Input: part model. Units: mm. Frame: model coordinates. A direction names the side the tool comes from. Give positions to 0.01 mm unless a question says otherwise; leave off trailing zeros. Write each loop counter-clockwise with the first axis right and the second up, starting at its lowest first coordinate (ties: lowest second). Pieces come first, ordered by that corner, then holes. Notation, with made-up numbers: (22, 76) -> (60, 76) arc R17 cw to (60, 81) -> close; hole circle Ø4 at (-27.75, 52.5). An arc over 180 degrees is marked (long way). Return JSON: item names as keys, results as strings. Group by question number.
Item 1: Line query: line 1 (Y direction, x = 0, z = 90); line 2 (Y direction, x = 0, z = -3); line 3 (X direction, y = -0.5, z = 57.5) (3 decimals). Output: solid intervals per line, ascending. Write a range as [from, to].
Item 2: Pin query (flat end, axial travel): P1, Ø5, axis at x = 0, y = 0, coming from the +Z side; P2, Ø1.3, axis at x = 0.5, y = 20.5, coming from the +Z side; P3, Ø2, axis at x = 12.5, z = 47, coming from the +Y side; P4, Ø1.5, axis at y = -4.5, z = 69, coming from the +X side. Return the tip coordinate at first contact, or that it passes through.
Item 3: Section B-B, the plane y = 0. Return loops of the section in (x, z).
Item 4: Mould query, pull axis Y, two halves, no side actions, for faces 3 (the face through (23.846, -7.509, 45.345)), 4 (the face through (0, 5, -5)), 5 (the face through (17, -10, 76.3)). Classes: released by +Y, released by -Y, zero draft, split by the parting line, or undercut.
Item 5: Section A-A, the plane x = 0. Return loops of the section in (y, z), then the cut area to 3 significant figures.
Item 6: Section C-C, the plane y = 20. Return loops of the section in (x, z).
Item 7: Set-up query: faces 1 (the face through (1.43, 2.75, -2.54)), 2 (the face through (-17, 10, 76.3)). Return all of +Z, -Z, +X, -X, +Y, -Y with unobstructed straight access to the full face (end or side cutting, diameter ignored); none if empty.
Item 8: Section D-D, the plane z = 62.5. Return loops of the section in (x, y), then the cut area to 3 significant figures.
from build123d import *

# Parameters (mm, degrees)
F0_R     = 25
F0_R_2   = 15
F1_DEPTH = 94.3
F2_R     = 2.25
F3_DEPTH = 18
F4_R     = 25
F5_DEPTH = 5
F6_R     = 3.1
F7_DEPTH = 25


with BuildPart() as f1:
    # F0 (on Top) → F1 (new body)
    with BuildSketch(Plane.XY):
        Circle(F0_R)
        Circle(F0_R_2, mode=Mode.SUBTRACT)
    extrude(amount=F1_DEPTH)

    # F2 (on face) → F3 (cut)
    with BuildSketch(Plane.XY.offset(94.3)):
        with Locations((0, 20)):
            Circle(F2_R)
        with Locations((-17.320508, -10)):
            Circle(F2_R)
        with Locations((17.320508, -10)):
            Circle(F2_R)
        with Locations((0, -20)):
            Circle(F2_R)
        with Locations((17.320508, 10)):
            Circle(F2_R)
        with Locations((-17.320508, 10)):
            Circle(F2_R)
    extrude(amount=-F3_DEPTH, mode=Mode.SUBTRACT)

    # F4 (on face) → F5 (join)
    with BuildSketch(Plane(origin=(0, 0, 0), x_dir=(1, 0, 0), z_dir=(0, 0, -1))):
        Circle(F4_R)
    extrude(amount=F5_DEPTH)

    # F6 (on face) → F7 (cut)
    with BuildSketch(Plane(origin=(0, 0, -5), x_dir=(1, 0, 0), z_dir=(0, 0, -1))):
        Circle(F6_R)
    extrude(amount=-F7_DEPTH, mode=Mode.SUBTRACT)


solid = f1.part
Answer below:
{
 "1": {"line 1": "y = [-25, -22.25], [-17.75, -15], [15, 17.75], [22.25, 25]", "line 2": "y = [-25, -3.1], [3.1, 25]", "line 3": "x = [-24.995, -14.992], [14.992, 24.995]"},
 "2": {"P1": "passes through", "P2": "stops at z = 76.3", "P3": "stops at y = 22.2", "P4": "stops at x = 24.72"},
 "3": {"outline": "(-25, -5) -> (-3.1, -5) -> (-3.1, 0) -> (-15, 0) -> (-15, 94.3) -> (-25, 94.3) -> close; (3.1, -5) -> (25, -5) -> (25, 94.3) -> (15, 94.3) -> (15, 0) -> (3.1, 0) -> close"},
 "4": {"face 3": "split by the parting line", "face 4": "zero draft", "face 5": "undercut"},
 "5": {"outline": "(-25, -5) -> (-3.1, -5) -> (-3.1, 0) -> (-15, 0) -> (-15, 94.3) -> (-17.75, 94.3) -> (-17.75, 76.3) -> (-22.25, 76.3) -> (-22.25, 94.3) -> (-25, 94.3) -> close; (3.1, -5) -> (25, -5) -> (25, 94.3) -> (22.25, 94.3) -> (22.25, 76.3) -> (17.75, 76.3) -> (17.75, 94.3) -> (15, 94.3) -> (15, 0) -> (3.1, 0) -> close", "area": "1,940 mm2"},
 "6": {"outline": "(-15, -5) -> (15, -5) -> (15, 94.3) -> (2.25, 94.3) -> (2.25, 76.3) -> (-2.25, 76.3) -> (-2.25, 94.3) -> (-15, 94.3) -> close"},
 "7": {"face 1": "+Z, -Z", "face 2": "+Z"},
 "8": {"outline": "circle Ø50 at (0, 0); hole circle Ø30 at (0, 0)", "area": "1,260 mm2"}
}
